The figure shows three views and two pictorial views of one solid part (mm, origin at its lowest corner). Answer the questions. A direction names the side the tool comes from. Coordinates: 2 decimals unless noted, no trailing zeros. Order: outer loops, then holes, each group sorted by start corner. A loop starts at its lowest first (then second) coordinate and runs counter-clockwise, first axis right, second up. Notation, with made-up numbers: (81, 31) -> (95, 31) arc R5 cw to (95, 37) -> close; hole circle Ø1 at (45.5, -33). An arc over 180 degrees is marked (long way). Use one line per item in the form item = value.
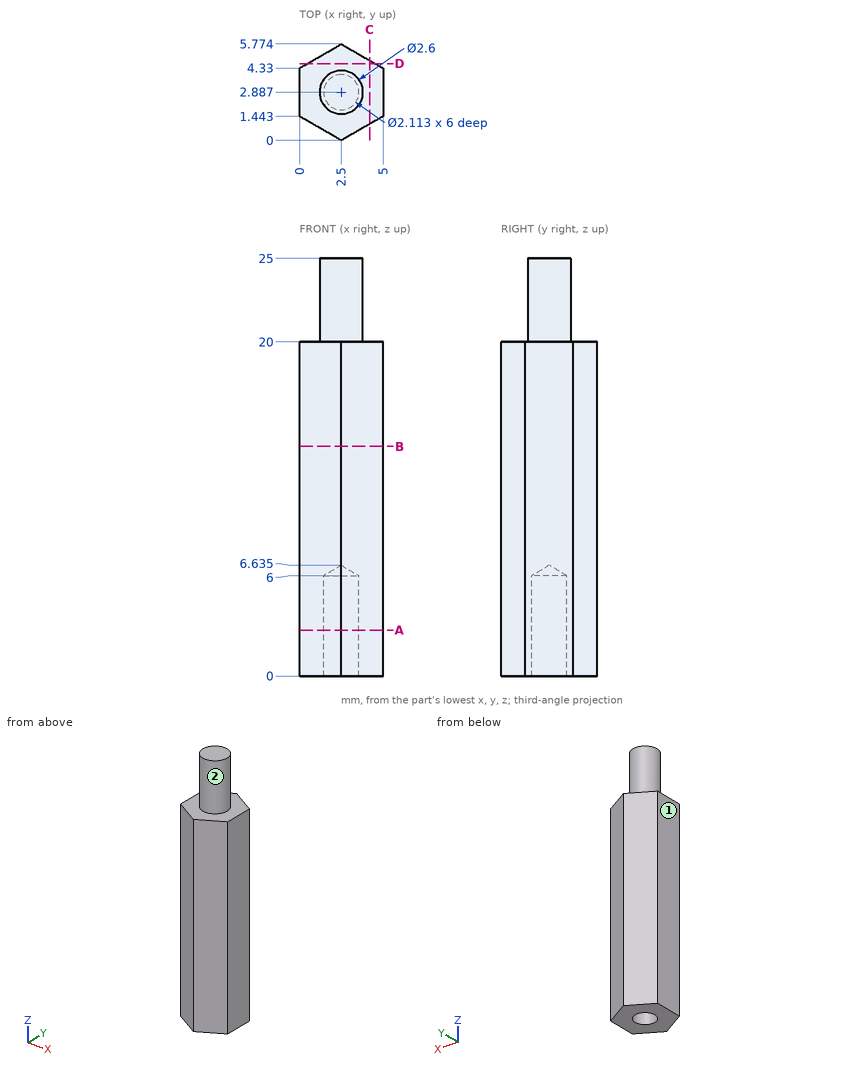
(1) This flat-tipped pin is pushed along its axis until it touches: P1, Ø1.7, axis at x = 2.5, y = 2.89, coming from the -Z side. Where does it stop, or does it pass through?
Data:
P1 = 6.12
(2) Section D-D on y = 4.6 is taken. Write down the section's boundary in (x, z), plus the area to 3 significant figures.
Data:
outline = (0.47, 0) -> (4.53, 0) -> (4.53, 20) -> (0.47, 20) -> close
area = 81.3 mm²
(3) Straight lines are drawn through the part: line 1 along Z through (x, y) = (4, 2.7); line 2 along Y through (x, z) = (2.2, 5.75) (1 decimal); line 3 along X through (y, z) = (3.5, 5). For each, find the intervals that lie inside material, in ascending order.
Data:
line_1 = 0 to 20
line_2 = 0.2 to 1.9, 3.9 to 5.6
line_3 = 0 to 1.64, 3.36 to 5
(4) Which of the six approach directions +Z, -Z, +X, -X, +Y, -Y give full straight-line access (tool end or side, diameter ignored) to the marked faces 1 and 2?
Data:
face_1 = +Z, -Z, -X, +Y, -Y
face_2 = +Z
(5) Section B-B on z = 13.75 is taken. Write down the section's boundary in (x, y).
Data:
outline = (0, 1.44) -> (2.5, 0) -> (5, 1.44) -> (5, 4.33) -> (2.5, 5.77) -> (0, 4.33) -> close
(6) Section C-C on x = 4.2 is taken. Write down the section's boundary in (y, z), plus the area to 3 significant figures.
Data:
outline = (0.98, 0) -> (4.79, 0) -> (4.79, 20) -> (0.98, 20) -> close
area = 76.2 mm²
(7) Section A-A on z = 2.75 is taken. Write down the section's boundary in (x, y).
Data:
outline = (0, 1.44) -> (2.5, 0) -> (5, 1.44) -> (5, 4.33) -> (2.5, 5.77) -> (0, 4.33) -> close; hole circle Ø2.11 at (2.5, 2.89)
